```python
from build123d import *

# Parameters (mm, degrees)
SKETCH_1_W           = 270
SKETCH_1_H           = 260
EXTRUDE_1_DEPTH      = 3
CUT_EXTRUDE_1_REACH  = 189.441
SKETCH_2_W           = 75
SKETCH_2_H           = 36
SKETCH_2_W_2         = 21
SKETCH_2_H_2         = 25
FILLET_1_R           = 5
SKETCH_3_R           = 1.5
CUT_EXTRUDE_2_DEPTH  = 10
SKETCH_4_R           = 1.5
CUT_EXTRUDE_3_DEPTH  = 188.440657276
SKETCH_5_R           = 1.5
CUT_EXTRUDE_4_DEPTH  = 188.440657276
SKETCH_6_R           = 1
CUT_EXTRUDE_5_DEPTH  = 188.440657276
SKETCH_7_R           = 1.5
CUT_EXTRUDE_6_DEPTH  = 188.440657276
SKETCH_8_R           = 1.5
CUT_EXTRUDE_7_DEPTH  = 188.440657276
SKETCH_9_R           = 1.1
CUT_EXTRUDE_8_DEPTH  = 188.440657276
CUT_EXTRUDE_9_REACH  = 189.441
SKETCH_10_R          = 1.5
SKETCH_11_R          = 12.5
CUT_EXTRUDE_10_DEPTH = 10


with BuildPart() as part:
    # 草图1 → 凸台-拉伸1 (new body)
    with BuildSketch(Plane.XY):
        Rectangle(SKETCH_1_W, SKETCH_1_H)
    extrude(amount=EXTRUDE_1_DEPTH)

    # 草图2 → 切除-拉伸1 (cut, up to next)
    with BuildSketch(Plane(origin=(0, 0, 0), x_dir=(-1, 0, 0), z_dir=(0, 0, -1)), mode=Mode.PRIVATE) as cut_extrude_1_sk1:
        with Locations((97.5, -112)):
            Rectangle(SKETCH_2_W, SKETCH_2_H)
    cut_extrude_1_tool1 = extrude(cut_extrude_1_sk1.sketch, amount=-CUT_EXTRUDE_1_REACH, mode=Mode.PRIVATE) & part.part
    # 草图2 → 切除-拉伸1 (cut, up to next)
    with BuildSketch(Plane(origin=(0, 0, 0), x_dir=(-1, 0, 0), z_dir=(0, 0, -1)), mode=Mode.PRIVATE) as cut_extrude_1_sk2:
        with Locations((97.25, -36)):
            Rectangle(SKETCH_2_W_2, SKETCH_2_H_2)
    cut_extrude_1_tool2 = extrude(cut_extrude_1_sk2.sketch, amount=-CUT_EXTRUDE_1_REACH, mode=Mode.PRIVATE) & part.part
    # 草图2 → 切除-拉伸1 (cut, up to next)
    with BuildSketch(Plane(origin=(0, 0, 0), x_dir=(-1, 0, 0), z_dir=(0, 0, -1)), mode=Mode.PRIVATE) as cut_extrude_1_sk3:
        with Locations((-97.5, 112)):
            Rectangle(SKETCH_2_W, SKETCH_2_H)
    cut_extrude_1_tool3 = extrude(cut_extrude_1_sk3.sketch, amount=-CUT_EXTRUDE_1_REACH, mode=Mode.PRIVATE) & part.part
    # 草图2 → 切除-拉伸1 (cut, up to next)
    with BuildSketch(Plane(origin=(0, 0, 0), x_dir=(-1, 0, 0), z_dir=(0, 0, -1)), mode=Mode.PRIVATE) as cut_extrude_1_sk4:
        with Locations((-97.25, -36)):
            Rectangle(SKETCH_2_W_2, SKETCH_2_H_2)
    cut_extrude_1_tool4 = extrude(cut_extrude_1_sk4.sketch, amount=-CUT_EXTRUDE_1_REACH, mode=Mode.PRIVATE) & part.part
    # 草图2 → 切除-拉伸1 (cut, up to next)
    with BuildSketch(Plane(origin=(0, 0, 0), x_dir=(-1, 0, 0), z_dir=(0, 0, -1)), mode=Mode.PRIVATE) as cut_extrude_1_sk5:
        with Locations((-97.5, -112)):
            Rectangle(SKETCH_2_W, SKETCH_2_H)
    cut_extrude_1_tool5 = extrude(cut_extrude_1_sk5.sketch, amount=-CUT_EXTRUDE_1_REACH, mode=Mode.PRIVATE) & part.part
    # 草图2 → 切除-拉伸1 (cut, up to next)
    with BuildSketch(Plane(origin=(0, 0, 0), x_dir=(-1, 0, 0), z_dir=(0, 0, -1)), mode=Mode.PRIVATE) as cut_extrude_1_sk6:
        with Locations((-97.25, 36)):
            Rectangle(SKETCH_2_W_2, SKETCH_2_H_2)
    cut_extrude_1_tool6 = extrude(cut_extrude_1_sk6.sketch, amount=-CUT_EXTRUDE_1_REACH, mode=Mode.PRIVATE) & part.part
    # 草图2 → 切除-拉伸1 (cut, up to next)
    with BuildSketch(Plane(origin=(0, 0, 0), x_dir=(-1, 0, 0), z_dir=(0, 0, -1)), mode=Mode.PRIVATE) as cut_extrude_1_sk7:
        with Locations((97.25, 36)):
            Rectangle(SKETCH_2_W_2, SKETCH_2_H_2)
    cut_extrude_1_tool7 = extrude(cut_extrude_1_sk7.sketch, amount=-CUT_EXTRUDE_1_REACH, mode=Mode.PRIVATE) & part.part
    # 草图2 → 切除-拉伸1 (cut, up to next)
    with BuildSketch(Plane(origin=(0, 0, 0), x_dir=(-1, 0, 0), z_dir=(0, 0, -1)), mode=Mode.PRIVATE) as cut_extrude_1_sk8:
        with Locations((97.5, 112)):
            Rectangle(SKETCH_2_W, SKETCH_2_H)
    cut_extrude_1_tool8 = extrude(cut_extrude_1_sk8.sketch, amount=-CUT_EXTRUDE_1_REACH, mode=Mode.PRIVATE) & part.part
    add(cut_extrude_1_tool1.solids().sort_by_distance((-97.5, -112, 0))[0], mode=Mode.SUBTRACT)
    add(cut_extrude_1_tool2.solids().sort_by_distance((-97.25, -36, 0))[0], mode=Mode.SUBTRACT)
    add(cut_extrude_1_tool3.solids().sort_by_distance((97.5, 112, 0))[0], mode=Mode.SUBTRACT)
    add(cut_extrude_1_tool4.solids().sort_by_distance((97.25, -36, 0))[0], mode=Mode.SUBTRACT)
    add(cut_extrude_1_tool5.solids().sort_by_distance((97.5, -112, 0))[0], mode=Mode.SUBTRACT)
    add(cut_extrude_1_tool6.solids().sort_by_distance((97.25, 36, 0))[0], mode=Mode.SUBTRACT)
    add(cut_extrude_1_tool7.solids().sort_by_distance((-97.25, 36, 0))[0], mode=Mode.SUBTRACT)
    add(cut_extrude_1_tool8.solids().sort_by_distance((-97.5, 112, 0))[0], mode=Mode.SUBTRACT)

    # 圆角1
    fillet_1_edges = [part.edges().sort_by_distance(p)[0] for p in [
        (135, 94, 1.5),
        (60, 130, 1.5),
        (60, 94, 1.5),
        (60, -130, 1.5),
        (135, -94, 1.5),
        (60, -94, 1.5),
        (-60, 130, 1.5),
        (-135, 94, 1.5),
        (-60, 94, 1.5),
        (-135, -94, 1.5),
        (-60, -130, 1.5),
        (-60, -94, 1.5),
    ]]
    fillet(fillet_1_edges, radius=FILLET_1_R)

    # 草图3 → 切除-拉伸2 (cut)
    with BuildSketch(Plane.XY.offset(3)):
        with Locations((-47, -32)):
            Circle(SKETCH_3_R)
        with Locations((47, -32)):
            Circle(SKETCH_3_R)
        with Locations((47, 62)):
            Circle(SKETCH_3_R)
        with Locations((-47, 62)):
            Circle(SKETCH_3_R)
    extrude(amount=-CUT_EXTRUDE_2_DEPTH, mode=Mode.SUBTRACT)

    # 草图4 → 切除-拉伸3 (cut, through all)
    with BuildSketch(Plane.XY.offset(3)):
        with Locations((45, 115)):
            Circle(SKETCH_4_R)
        with Locations((120, 87)):
            Circle(SKETCH_4_R)
        with Locations((120, -87)):
            Circle(SKETCH_4_R)
        with Locations((45, -115)):
            Circle(SKETCH_4_R)
        with Locations(Location((-45, -115, 0), (0, 0, 180))):
            Circle(SKETCH_4_R)
        with Locations(Location((-120, -87, 0), (0, 0, 180))):
            Circle(SKETCH_4_R)
        with Locations(Location((-120, 87, 0), (0, 0, 180))):
            Circle(SKETCH_4_R)
        with Locations(Location((-45, 115, 0), (0, 0, 180))):
            Circle(SKETCH_4_R)
        with Locations((-65, 40)):
            Circle(SKETCH_4_R)
        with Locations((65, 40)):
            Circle(SKETCH_4_R)
        with Locations((-65, -40)):
            Circle(SKETCH_4_R)
        with Locations((65, -40)):
            Circle(SKETCH_4_R)
    extrude(amount=-CUT_EXTRUDE_3_DEPTH, mode=Mode.SUBTRACT)

    # 草图5 → 切除-拉伸4 (cut, through all)
    with BuildSketch(Plane.XY.offset(3)):
        with Locations((125.408441645, -45.5)):
            Circle(SKETCH_5_R)
        with Locations((125.406892783, -75.49999996)):
            Circle(SKETCH_5_R)
        with Locations(Location((125.406892783, 75.49999996, 0), (0, 0, 180))):
            Circle(SKETCH_5_R)
        with Locations(Location((125.408441645, 45.5, 0), (0, 0, 180))):
            Circle(SKETCH_5_R)
        with Locations(Location((-125.406892783, -75.49999996, 0), (0, 0, 180))):
            Circle(SKETCH_5_R)
        with Locations(Location((-125.408441645, -45.5, 0), (0, 0, 180))):
            Circle(SKETCH_5_R)
        with Locations((-125.408441645, 45.5)):
            Circle(SKETCH_5_R)
        with Locations((-125.406892783, 75.49999996)):
            Circle(SKETCH_5_R)
    extrude(amount=-CUT_EXTRUDE_4_DEPTH, mode=Mode.SUBTRACT)

    # 草图6 → 切除-拉伸5 (cut, through all)
    with BuildSketch(Plane.XY.offset(3)):
        with Locations((-6, -114.75)):
            Circle(SKETCH_6_R)
        with Locations((6, -114.75)):
            Circle(SKETCH_6_R)
        with Locations((-6, -122.75)):
            Circle(SKETCH_6_R)
        with Locations((6, -122.75)):
            Circle(SKETCH_6_R)
        with Locations((-6, -72.75)):
            Circle(SKETCH_6_R)
        with Locations((6, -72.75)):
            Circle(SKETCH_6_R)
        with Locations((-6, -64.75)):
            Circle(SKETCH_6_R)
        with Locations((6, -64.75)):
            Circle(SKETCH_6_R)
    extrude(amount=-CUT_EXTRUDE_5_DEPTH, mode=Mode.SUBTRACT)

    # 草图7 → 切除-拉伸6 (cut, through all)
    with BuildSketch(Plane.XY.offset(3)):
        with Locations((110.9, 10.5)):
            Circle(SKETCH_7_R)
        with Locations((110.9, -10.5)):
            Circle(SKETCH_7_R)
    extrude(amount=-CUT_EXTRUDE_6_DEPTH, mode=Mode.SUBTRACT)

    # 草图8 → 切除-拉伸7 (cut, through all)
    with BuildSketch(Plane.XY.offset(3)):
        with Locations((-40, 124)):
            Circle(SKETCH_8_R)
        with Locations((40, 124)):
            Circle(SKETCH_8_R)
    extrude(amount=-CUT_EXTRUDE_7_DEPTH, mode=Mode.SUBTRACT)

    # 草图9 → 切除-拉伸8 (cut, through all)
    with BuildSketch(Plane.XY.offset(3)):
        with Locations((-13, 119)):
            Circle(SKETCH_9_R)
        with Locations((13, 119)):
            Circle(SKETCH_9_R)
        with Locations((-13, 95)):
            Circle(SKETCH_9_R)
        with Locations((13, 95)):
            Circle(SKETCH_9_R)
    extrude(amount=-CUT_EXTRUDE_8_DEPTH, mode=Mode.SUBTRACT)

    # 草图10 → 切除-拉伸9 (cut, up to next)
    with BuildSketch(Plane.XY.offset(3), mode=Mode.PRIVATE) as cut_extrude_9_sk1:
        with Locations((-44.249999943, 85.000444876)):
            Circle(SKETCH_10_R)
    cut_extrude_9_tool1 = extrude(cut_extrude_9_sk1.sketch, amount=-CUT_EXTRUDE_9_REACH, mode=Mode.PRIVATE) & part.part
    # 草图10 → 切除-拉伸9 (cut, up to next)
    with BuildSketch(Plane.XY.offset(3), mode=Mode.PRIVATE) as cut_extrude_9_sk2:
        with Locations((-44.249999943, 75)):
            Circle(SKETCH_10_R)
    cut_extrude_9_tool2 = extrude(cut_extrude_9_sk2.sketch, amount=-CUT_EXTRUDE_9_REACH, mode=Mode.PRIVATE) & part.part
    # 草图10 → 切除-拉伸9 (cut, up to next)
    with BuildSketch(Plane.XY.offset(3), mode=Mode.PRIVATE) as cut_extrude_9_sk3:
        with Locations((24.25, 85)):
            Circle(SKETCH_10_R)
    cut_extrude_9_tool3 = extrude(cut_extrude_9_sk3.sketch, amount=-CUT_EXTRUDE_9_REACH, mode=Mode.PRIVATE) & part.part
    # 草图10 → 切除-拉伸9 (cut, up to next)
    with BuildSketch(Plane.XY.offset(3), mode=Mode.PRIVATE) as cut_extrude_9_sk4:
        with Locations((24.25, 75)):
            Circle(SKETCH_10_R)
    cut_extrude_9_tool4 = extrude(cut_extrude_9_sk4.sketch, amount=-CUT_EXTRUDE_9_REACH, mode=Mode.PRIVATE) & part.part
    add(cut_extrude_9_tool1.solids().sort_by_distance((-44.25, 85.000445, 3))[0], mode=Mode.SUBTRACT)
    add(cut_extrude_9_tool2.solids().sort_by_distance((-44.25, 75, 3))[0], mode=Mode.SUBTRACT)
    add(cut_extrude_9_tool3.solids().sort_by_distance((24.25, 85, 3))[0], mode=Mode.SUBTRACT)
    add(cut_extrude_9_tool4.solids().sort_by_distance((24.25, 75, 3))[0], mode=Mode.SUBTRACT)

    # 草图11 → 切除-拉伸10 (cut)
    with BuildSketch(Plane.XY.offset(3)):
        with Locations((45, -60)):
            Circle(SKETCH_11_R)
    extrude(amount=-CUT_EXTRUDE_10_DEPTH, mode=Mode.SUBTRACT)


solid = part.part
```
CAD build for the part. Positions are in the model's coordinates, mm. Round coordinates to 2 decimals unless told otherwise and drop trailing zeros. Order: outer loops, then holes, each group sorted by start corner. A loop starts at its lowest first (then second) coordinate and runs counter-clockwise, first axis right, second up. Notation, with made-up numbers: (60.5, -24) - (77.5, -24) arc R14 cw to (77.5, -17) - close; hole circle Ø8 at (-34, 42). An arc over 180 degrees is marked (long way). Use CSV: the item, a comma, the result in double quotes. Start each with the question number.
1) Wall check: L1, parallel to Y at x = 13, z = 2.3; L2, parallel to X at y = 115, z = 0.7; L3, parallel to X at y = -122.75, z = 0.8. Give the ranges that are in metal, low to high. Write a range as [from, to].
2) Saw through at B-B (z = 1.8). Count the separate pieces of the cut face and the enclosed holes in it, and give its area (3 significant figures).
3) Pin check, flat tips, straight feed: pin 1 Ø1.8 at (x, y) = (-6, -72.75) entering from +Z; pin 2 Ø0.9 at (x, z) = (93.5, 1.5) entering from +Y; pin 3 Ø0.9 at (y, z) = (-107, 2) entering from +X; pin 4 Ø1 at (x, z) = (-62.5, 1.5) entering from +Y. Stop position of each tip, or through.
4) Two-plate mould, pull along X, no slides. Class faces 1 (the flat face through (-2, 2, 0)), 2 (the cylindrical face through (35.79, -51.55, 1.52)): pulls with the +X half, pulls with the -X half, needs draft (parallel to the pull), parting line crosses it, or undercut.
5) Saw through at A-A (x = -97). List the corners of the cut face in (y, z), and give its area (3 significant figures).
Values follow:
1,L1,"y = [-130, 93.9], [96.1, 117.9], [120.1, 130]"
1,L2,"x = [-60, -46.5], [-43.5, 43.5], [46.5, 60]"
1,L3,"x = [-60, -7], [-5, 5], [7, 60]"
2,separate pieces,"1"
2,enclosed holes,"49"
2,area,"56,500 mm2"
3,pin 1,"passes through"
3,pin 2,"stops at y = 94"
3,pin 3,"stops at x = 60"
3,pin 4,"stops at y = 95"
4,face 1,"needs draft"
4,face 2,"undercut"
5,outline,"(-94, 0) - (-48.5, 0) - (-48.5, 3) - (-94, 3) - close; (-23.5, 0) - (23.5, 0) - (23.5, 3) - (-23.5, 3) - close; (48.5, 0) - (94, 0) - (94, 3) - (48.5, 3) - close"
5,area,"414 mm2"
